Autodesk Inventor part; units mm, degrees
ref_plane "YZ Plane" through (0, 0, 0) normal (1, 0, 0) x (0, 1, 0)
ref_plane "XZ Plane" through (0, 0, 0) normal (0, 1, 0) x (-1, 0, 0)
ref_plane "XY Plane" through (0, 0, 0) normal (0, 0, 1) x (1, 0, 0)
sketch "Sketch1" plane through (0, 0, 0) normal (0, 1, 0) x (-1, 0, 0)
  line L0 (3.175, 0) -> (187.325, 0)
  line L1 (187.325, -196.85) -> (3.175, -196.85)
  line L2 (111.2012, -7.145) -> (111.2012, -12.7)
  line L3 (111.2012, -12.7) -> (123.9012, -12.7)
  line L4 (123.9012, -12.7) -> (123.9012, -7.145)
  line L5 (79.2988, -7.1374) -> (79.2988, -12.7)
  line L6 (79.2988, -12.7) -> (66.5988, -12.7)
  line L7 (66.5988, -12.7) -> (66.5988, -7.1374)
  line L8 (66.5988, -88.9) -> (79.2988, -88.9)
  line L9 (79.2988, -88.9) -> (79.2988, -83.3374)
  line L10 (66.5988, -83.3374) -> (66.5988, -88.9)
  line L11 (123.9012, -88.9) -> (111.2012, -88.9)
  line L12 (111.2012, -88.9) -> (111.2012, -83.3374)
  line L13 (123.9012, -83.3374) -> (123.9012, -88.9)
  line L14 (190.5, -25.4) -> (193.675, -25.4)
  line L15 (193.675, -63.5) -> (190.5, -63.5)
  line L16 (0, -25.4) -> (-3.175, -25.4)
  line L17 (-3.175, -63.5) -> (0, -63.5)
  line L18 (190.5, -171.45) -> (193.675, -171.45)
  line L19 (193.675, -133.35) -> (190.5, -133.35)
  line L20 (0, -171.45) -> (-3.175, -171.45)
  line L21 (-3.175, -133.35) -> (0, -133.35)
  line L22 (190.5, -171.45) -> (193.675, -171.45)
  line L23 (190.5, -25.4) -> (187.325, -25.4)
  line L24 (190.5, -63.5) -> (187.325, -63.5)
  line L25 (190.5, -133.35) -> (187.325, -133.35)
  line L26 (190.5, -171.45) -> (187.325, -171.45)
  line L27 (193.675, -25.4) -> (193.675, -63.5)
  line L28 (193.675, -133.35) -> (193.675, -171.45)
  line L29 (187.325, -171.45) -> (187.325, -196.85)
  line L30 (187.325, 0) -> (187.325, -25.4)
  line L31 (187.325, -63.5) -> (187.325, -133.35)
  line L32 (0, -171.45) -> (3.175, -171.45)
  line L33 (0, -133.35) -> (3.175, -133.35)
  line L34 (0, -63.5) -> (3.175, -63.5)
  line L35 (0, -25.4) -> (3.175, -25.4)
  line L36 (-3.175, -25.4) -> (-3.175, -63.5)
  line L37 (-3.175, -133.35) -> (-3.175, -171.45)
  line L38 (3.175, 0) -> (3.175, -25.4)
  line L39 (3.175, -63.5) -> (3.175, -133.35)
  line L40 (3.175, -171.45) -> (3.175, -196.85)
  line L41 (123.9012, -12.7) -> (111.2012, -12.7)
  line L42 (111.2012, -12.7) -> (111.2012, -7.145)
  line L43 (111.2012, -7.145) -> (123.9012, -7.145)
  line L44 (123.9012, -7.145) -> (123.9012, -12.7)
  line L45 (123.9012, -88.9) -> (111.2012, -88.9)
  line L46 (111.2012, -88.9) -> (111.2012, -83.3374)
  line L47 (111.2012, -83.3374) -> (123.9012, -83.3374)
  line L48 (123.9012, -83.3374) -> (123.9012, -88.9)
  line L49 (79.2988, -12.7) -> (66.5988, -12.7)
  line L50 (66.5988, -12.7) -> (66.5988, -7.1374)
  line L51 (66.5988, -7.1374) -> (79.2988, -7.1374)
  line L52 (79.2988, -7.1374) -> (79.2988, -12.7)
  line L53 (79.2988, -88.9) -> (66.5988, -88.9)
  line L54 (66.5988, -88.9) -> (66.5988, -83.3374)
  line L55 (66.5988, -83.3374) -> (79.2988, -83.3374)
  line L56 (79.2988, -83.3374) -> (79.2988, -88.9)
  point P0 (0, 0)
  dimension "d4" = 12.7
  dimension "d6" = 12.7
  dimension "d29" = 5.555
  dimension "d31" = 5.5626
extrude "Extrusion1" add sketch "Sketch1" along normal blind 5.5563
sketch "Sketch2" plane through (0, 5.5563, 0) normal (0, 1, 0) x (1, 0, 0)
  circle A0 centre (-39.6875, 144.4625) radius 12.7
  point P0 (0, 0)
extrude "Extrusion2" cut sketch "Sketch2" against normal blind 6.35
properties part number "mid_floor"
Geometry check sheet. Reference: the model listing, model coordinates, mm. A direction names the side the tool comes from. Round coordinates to 2 decimals unless told otherwise and drop trailing zeros. Order: outer loops, then holes, each group sorted by start corner. A loop starts at its lowest first (then second) coordinate and runs counter-clockwise, first axis right, second up. Notation, with made-up numbers: (81, 73.5) -> (121, 73.5) arc R30 ccw to (121, 95.5) -> close; hole circle Ø8 at (5.25, 57). An arc over 180 degrees is marked (long way). Use one line per item in the form item = value.
1. Cross-section at A-A, the plane z = -148. Enter the section's corners in (x, y) (3 decimals).
Working result:
outline = (-193.675, 0) -> (-51.885, 0) -> (-51.885, 5.556) -> (-193.675, 5.556) -> close; (-27.49, 0) -> (3.175, 0) -> (3.175, 5.556) -> (-27.49, 5.556) -> close
2. Go/stop test with flat-tipped pins: pin 1 (1.7 mm diameter, centred on y = 3, z = -17.5, fed in from +X) (3 decimals); pin 2 (1.7 mm diameter, centred on y = 2.5, z = -86.5, fed in from -X) (3 decimals); pin 3 (23 mm diameter, centred on x = -39.69, z = -144.46, fed in from +Y). Record where each tip stops, or that it passes through.
Working result:
pin_1 = -3.175
pin_2 = -187.325
pin_3 = through
3. Scan lines: line 1 along X through (y, z) = (0.85, -9.5) (3 decimals); line 2 along Z through (x, y) = (-123, 2.35) (3 decimals); line 3 along X through (y, z) = (5, -180) (3 decimals). Record each from-to range of solid material in increasing order. Write a range as from..to.
Working result:
line_1 = -187.325..-123.901, -111.201..-79.299, -66.599..-3.175
line_2 = -196.85..-88.9, -83.337..-12.7, -7.145..0
line_3 = -187.325..-3.175
4. Cross-section at C-C, the plane y = 2.75. Count the separate pieces of the cut face and the enclosed holes in it, plus the area to 3 significant figures.
Working result:
separate_pieces = 1
enclosed_holes = 5
area = 36,400 mm^2
5. Mould release check, pull along Z, two halves, no side actions. Record for faces 6 (the face through (0, 3, -171.45)), 7 (the face through (0, 3, -133.35)), 8 (the face through (-94, 0, -97)), 9 (the face through (-94, 3, 0)): pulls with the +Z half, pulls with the -Z half, needs draft (parallel to the pull), parting line crosses it, or undercut.
Working result:
face_6 = pulls with the -Z half
face_7 = undercut
face_8 = needs draft
face_9 = pulls with the +Z half
6. Set-up check for faces 1 (the face through (-187.325, 3, -184)), 2 (the face through (-94, 5.556, -97)), 3 (the face through (-191, 3, -63.5)), 4 (the face through (-66.599, 3, -10)), 5 (the face through (-3.175, 3, -184)): record each of +Z, -Z, +X, -X, +Y, -Y from which the full face is reachable in a straight line by a thin tool's end or side.
Working result:
face_1 = -Z, -X, +Y, -Y
face_2 = +Z, -Z, +X, -X, +Y
face_3 = -X, +Y, -Y
face_4 = +Y, -Y
face_5 = -Z, +X, +Y, -Y
7. Cross-section at B-B, the plane z = -106. Enter the section's corners in (x, y) (3 decimals), plus the area to 3 significant figures.
Working result:
outline = (-187.325, 0) -> (-3.175, 0) -> (-3.175, 5.556) -> (-187.325, 5.556) -> close
area = 1,020 mm^2
